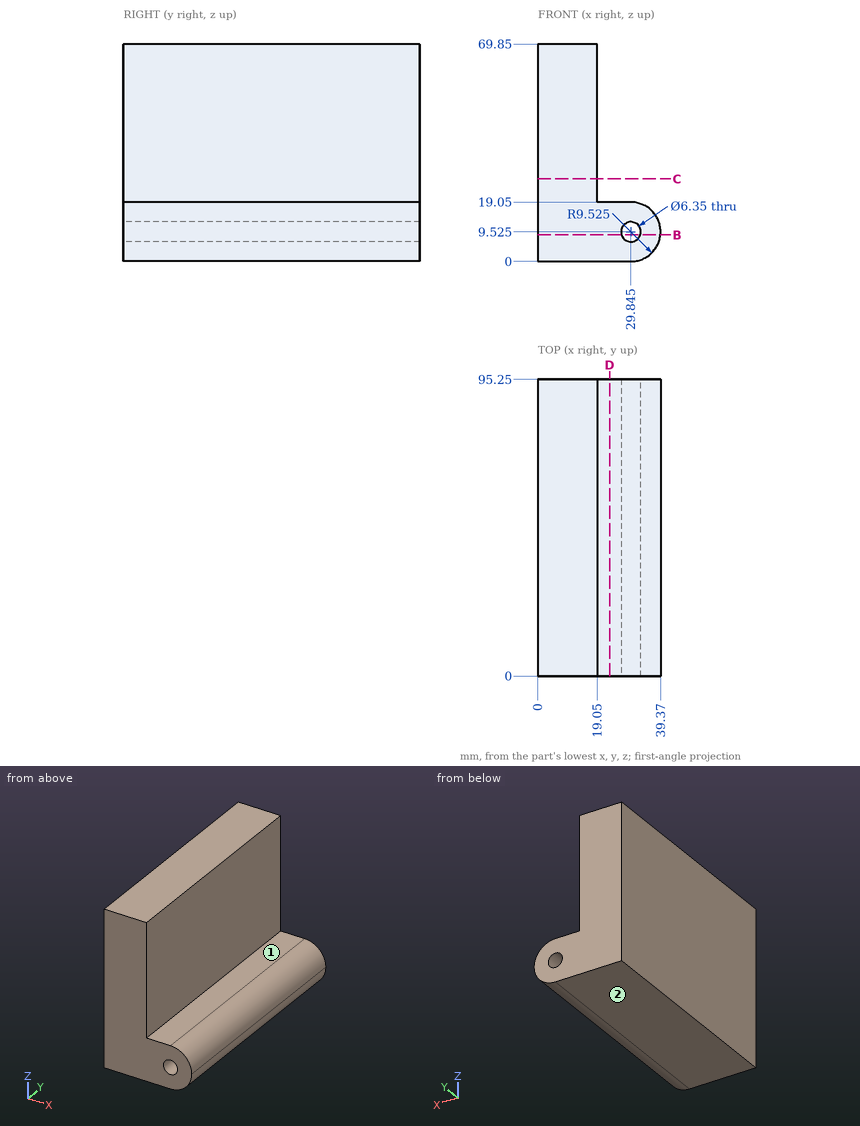
Drawing for the job (mm, zero at the part's lowest x, y, z). A direction names the side the tool comes from. Round coordinates to 2 decimals unless told otherwise and drop trailing zeros. Loops run counter-clockwise (first coordinate to the right, second up) from the corner with the lowest first, then second, coordinate; pieces in that order, holes last. Notation, with made-up numbers: (35, 83.5) - (89, 83.5) arc R18 ccw to (89, 110.5) - close; hole circle Ø10 at (15.5, 87). An arc over 180 degrees is marked (long way). Return JSON: item names as keys, results as strings. Group by question number.
Q1. Band-saw the part on D-D on x = 23. Give the cut face in (y, z), plus the area to 3 significant figures.
Q2. Drill centre line: line 1 along Z through (x, y) = (21.5, 84.5). Where is it in solid material? Low to high. Write a range as [from, to].
Q3. Flat gauge pins, fed straight in: pin 1 Ø2 at (x, y) = (24.5, 60) entering from -Z; pin 2 Ø12 at (x, y) = (26.5, 25.5) entering from +Z. Where does each tip first touch, or does it go through?
Q4. Band-saw the part on C-C on z = 26.5. Give the cut face in (x, y), plus the area to 3 significant figures.
Q5. Band-saw the part on B-B on z = 8.5. Give the cut face in (x, y).
Q6. Tool access for the marked faces 1 and 2: list every direction of +Z, -Z, +X, -X, +Y, -Y with a clear straight run to the whole face (end or side of a thin tool).
Solutions:
{
 "1": {"outline": "(0, 0) - (95.25, 0) - (95.25, 19.05) - (0, 19.05) - close", "area": "1,810 mm^2"},
 "2": {"line 1": "z = [0, 19.05]"},
 "3": {"pin 1": "stops at z = 0", "pin 2": "stops at z = 19.05"},
 "4": {"outline": "(0, 0) - (19.05, 0) - (19.05, 95.25) - (0, 95.25) - close", "area": "1,810 mm^2"},
 "5": {"outline": "(0, 0) - (26.84, 0) - (26.84, 95.25) - (0, 95.25) - close; (32.85, 0) - (39.31, 0) - (39.31, 95.25) - (32.85, 95.25) - close"},
 "6": {"face 1": "+Z, +X, +Y, -Y", "face 2": "-Z, +X, -X, +Y, -Y"}
}
